from build123d import *

# Parameters (mm, degrees)
F1_DEPTH = 85
F2_R     = 2.25
F3_DEPTH = 50
F4_R     = 2.25
F5_DEPTH = 25
F6_W     = 7.057262
F6_H     = 25
F7_DEPTH = 85


with BuildPart() as f1:
    # F0 (on Top) → F1 (new body)
    with BuildSketch(Plane.XY):
        Polygon((-30.368601, 20.967192), (-30.368601, 15.967192), (-15.368601, 15.967192), (-15.368601, 8.098098), (-30.368601, 8.098098), (-30.368601, -1.901902), (9.631399, -1.901902), (9.631399, 70.967192), (-4.483124, 70.967192), (-4.483124, 20.967192), align=None)
    extrude(amount=F1_DEPTH)

    # F2 (on face) → F3 (cut)
    with BuildSketch(Plane(origin=(0, 20.967192, 0), x_dir=(-1, 0, 0), z_dir=(0, 1, 0))):
        with Locations((25.368601, 8)):
            Circle(F2_R)
        with Locations((25.368601, 78)):
            Circle(F2_R)
    extrude(amount=-F3_DEPTH, mode=Mode.SUBTRACT)

    # F4 (on face) → F5 (cut)
    with BuildSketch(Plane(origin=(-4.483124, 0, 0), x_dir=(0, -1, 0), z_dir=(-1, 0, 0))):
        with BuildLine():
            Line((-70.967192, 65), (-70.967192, 20))
            Line((-70.967192, 20), (-40.967192, 20))
            ThreePointArc((-40.967192, 20), (-30.36059, 24.393398), (-25.967192, 35))
            Line((-25.967192, 35), (-25.967192, 50))
            ThreePointArc((-25.967192, 50), (-30.36059, 60.606602), (-40.967192, 65))
            Line((-40.967192, 65), (-70.967192, 65))
        make_face()
        with Locations((-60.967192, 75)):
            Circle(F4_R)
        with Locations((-60.967192, 10)):
            Circle(F4_R)
    extrude(amount=-F5_DEPTH, mode=Mode.SUBTRACT)

    # F6 (on face) → F7 (cut)
    with BuildSketch(Plane.XY.offset(85)):
        with Locations((6.102768, 58.467192)):
            Rectangle(F6_W, F6_H)
    extrude(amount=-F7_DEPTH, mode=Mode.SUBTRACT)


solid = f1.part
Input: part model. Units: mm. Frame: model coordinates. A direction names the side the tool comes from. Give positions to 0.01 mm unless a question says otherwise; leave off trailing zeros. Write each loop counter-clockwise with the first axis right and the second up, starting at its lowest first coordinate (ties: lowest second). Pieces come first, ordered by that corner, then holes.
Q1. Section A-A, the plane y = 43. Output: boundary loops of the cut face in (x, z).
Q2. Section D-D, the plane x = 5.5. Output: boundary loops of the cut face in (y, z), plus the area to 3 significant figures.
Q3. First-contact query: P1, Ø16, axis at y = 62.5, z = 7.5, coming from the +X side; P2, Ø7, axis at x = -0.5, z = 39, coming from the +Y side; P3, Ø8, axis at x = -12, z = 50.5, coming from the +Y side. Flat tips, straight axial feed; report the tip coordinate or a pass-through.
Q4. Material intervals for probe 1 along Y at (x, z) = (-18, 59.5); probe 2 along Y at (x, z) = (7, 71); probe 3 along Y at (x, z) = (-9, 18), sorted ascending.
Q5. Section B-B, the plane x = -20. Output: boundary loops of the cut face in (y, z), plus the area to 4 significant figures.
Q6. Section C-C, the plane z = 30.5. Output: boundary loops of the cut face in (x, y), plus the area to 3 significant figures.
Q7. Set-up query: faces 4 (the face through (-23, 8.098, 42)), 5 (the face through (-24.9, 3.2, 75.8)), 6 (the face through (-4.483, 24, 42)), 7 (the face through (2.475, 30.245, 60.489)), 8 (the face through (6, 45.967, 10)). Return all of +Z, -Z, +X, -X, +Y, -Y with unobstructed straight access to the full face (end or side cutting, diameter ignored); none if empty.
Q8. Pull-direction query (Z, two-part tool) for faces 1 (the face through (-6, 19, 0)), 2 (the face through (-1, 56, 20)), 3 (the face through (-23, 15.967, 42)); classes: pulls with the +Z half, pulls with the -Z half, needs draft (parallel to the pull), parting line crosses it, or undercut.
Filled in:
1. outline: (-4.48, 0) - (9.63, 0) - (9.63, 20) - (-4.48, 20) - close; (-4.48, 65) - (9.63, 65) - (9.63, 85) - (-4.48, 85) - close
2. outline: (-1.9, 0) - (45.97, 0) - (45.97, 20) - (40.97, 20) arc R15 cw to (25.97, 35) - (25.97, 50) arc R15 cw to (40.97, 65) - (45.97, 65) - (45.97, 85) - (-1.9, 85) - close
2. area: 3,270 mm2
3. P1: stops at x = 2.57
3. P2: stops at y = 25.97
3. P3: stops at y = 20.97
4. probe 1: y = -1.9 to 8.1, 15.97 to 20.97
4. probe 2: y = -1.9 to 45.97
4. probe 3: y = -1.9 to 20.97
5. outline: (-1.9, 0) - (8.1, 0) - (8.1, 85) - (-1.9, 85) - close; (15.97, 0) - (20.97, 0) - (20.97, 85) - (15.97, 85) - close
5. area: 1,275 mm2
6. outline: (-30.37, -1.9) - (9.63, -1.9) - (9.63, 26.66) - (-4.48, 26.66) - (-4.48, 20.97) - (-30.37, 20.97) - (-30.37, 15.97) - (-15.37, 15.97) - (-15.37, 8.1) - (-30.37, 8.1) - close
6. area: 877 mm2
7. face 4: +Z, -Z, -X
7. face 5: +Y, -Y
7. face 6: +Z, -Z, -X, +Y
7. face 7: +X, -X, +Y
7. face 8: +Z, -Z, +X, +Y
8. face 1: pulls with the -Z half
8. face 2: undercut
8. face 3: needs draft
